Study the drawing (mm; zero at the part's minimum x, y, z) and answer. A direction names the side the tool comes from. Give positions to 0.01 mm unless a question says otherwise; leave off trailing zeros. Order: outer loops, then holes, each group sorted by start corner. A loop starts at its lowest first (then second) coordinate and runs counter-clockwise, first axis right, second up. Notation, with made-up numbers: (80, 61.25) - (122, 61.25) arc R14 cw to (122, 80.25) - close; hole circle Ø8 at (0, 22). An arc over 180 degrees is marked (long way). Write each question's results on one line, items separated by ' | '. Start each with the question number.
1. Section C-C (x = 7.75) is taken. Give the vertices of the cut face in (y, z) (1 decimal).
2. Section D-D (x = 10.75) is taken. Give the vertices of the cut face in (y, z) (1 decimal).
3. Section A-A (y = 4.45) is taken. Give the vertices of the cut face in (x, z) (1 decimal).
4. Which of the six approach directions +Z, -Z, +X, -X, +Y, -Y give full straight-line access (tool end or side, diameter ignored) to the marked faces 4, 5 and 6?
5. Flat-ended cylindrical pins translate along their axes: pin 1 (2 mm diameter, centred on x = 10.5, y = 3, fed in from -Z); pin 2 (1.1 mm diameter, centred on y = 4.5, z = 4, fed in from +X); pin 3 (0.5 mm diameter, centred on y = 5, z = 3.5, fed in from -X). Find the tip coordinate at first contact, or state that the pin passes through.
6. Find the intervals of material crossed by L1, parallel to Y at x = 10, z = 0.75 (1 decimal); L2, parallel to X at y = 0.5, z = 3.25; L3, parallel to Z at x = 5, y = 3.7 (1 decimal), in increasing order.
7. Determine the mould class of the marked faces 1, 2 and 3 for opening direction Z: released by +Z, released by -Z, zero draft, split by the parting line, or undercut.
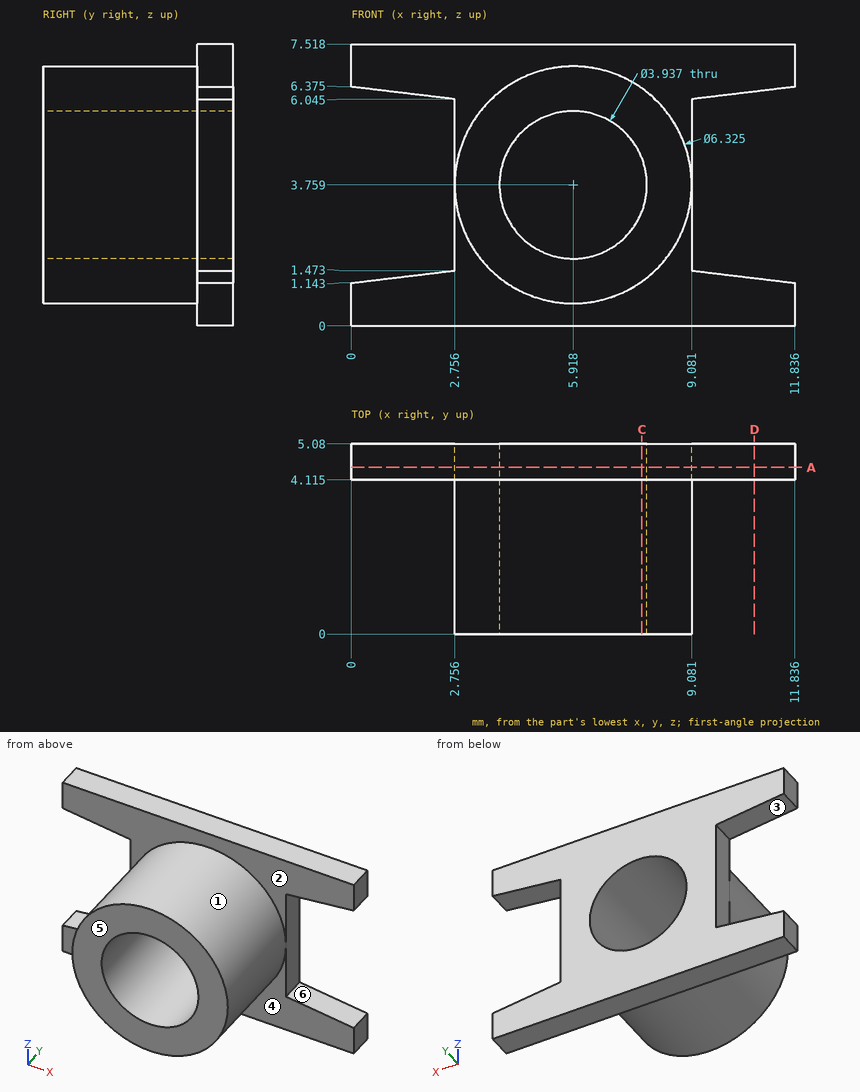
Reported:
1) outline: (0, 1.2) - (4.1, 1.2) - (4.1, 0) - (5.1, 0) - (5.1, 3) - (0, 3) - close; (0, 4.5) - (5.1, 4.5) - (5.1, 7.5) - (4.1, 7.5) - (4.1, 6.3) - (0, 6.3) - close
2) outline: (4.1, 0) - (5.1, 0) - (5.1, 1.3) - (4.1, 1.3) - close; (4.1, 6.2) - (5.1, 6.2) - (5.1, 7.5) - (4.1, 7.5) - close
3) outline: (0, 0) - (11.8, 0) - (11.8, 1.1) - (9.1, 1.5) - (9.1, 6) - (11.8, 6.4) - (11.8, 7.5) - (0, 7.5) - (0, 6.4) - (2.8, 6) - (2.8, 1.5) - (0, 1.1) - close; hole circle Ø3.9 at (5.9, 3.8)
4) face 4: -Z, -Y | face 5: +Z, -Z, +X, -X, -Y | face 6: +X, +Y, -Y
5) pin 1: through | pin 2: x = 9.08 | pin 3: x = 2.76
6) L1: 4.1 to 5.1 | L2: 2.8 to 4.02, 7.82 to 9.04 | L3: 0.7 to 2, 5.5 to 6.8
7) face 1: split by the parting line | face 2: zero draft | face 3: undercut
